Geometry check sheet. Reference: the model listing, model coordinates, mm. A direction names the side the tool comes from. Round coordinates to 2 decimals unless told otherwise and drop trailing zeros. Loops run counter-clockwise (first coordinate to the right, second up) from the corner with the lowest first, then second, coordinate; pieces in that order, holes last. Notation, with made-up numbers: M 63.25,23.5 L 115.25,23.5 A24 cw 115.25,56.5 Z; hole C 74.5,-22.75 d1. An arc over 180 degrees is marked long. Write item = value, one per line.
from build123d import *

# Parameters (mm, degrees)
SKETCH1_W           = 20
SKETCH1_H           = 20
BOSS_EXTRUDE1_DEPTH = 150
SKETCH3_R           = 9
BOSS_EXTRUDE2_DEPTH = 100
SKETCH2_R           = 7.5
BOSS_EXTRUDE3_DEPTH = 150
SKETCH7_R           = 0.25
BOSS_EXTRUDE4_DEPTH = 10
SKETCH8_R           = 2.5
BOSS_EXTRUDE5_DEPTH = 0.5
SKETCH19_W          = 126.5
SKETCH19_H          = 0.1
BOSS_EXTRUDE6_DEPTH = 0.5


with BuildPart() as part:
    # Sketch1 → Boss-Extrude1 (new body)
    with BuildSketch(Plane.XY):
        Rectangle(SKETCH1_W, SKETCH1_H)
    extrude(amount=BOSS_EXTRUDE1_DEPTH)

    # Sketch3 → Boss-Extrude2 (add)
    with BuildSketch(Plane.XZ.offset(10)):
        with Locations((0, 75)):
            Circle(SKETCH3_R)
    extrude(amount=BOSS_EXTRUDE2_DEPTH)

    # Sketch2 → Boss-Extrude3 (add)
    with BuildSketch(Plane(origin=(0, 10, 0), x_dir=(1, 0, 0), z_dir=(0, 1, 0))):
        with Locations((0, -12)):
            Circle(SKETCH2_R)
        with Locations((0, -138)):
            Circle(SKETCH2_R)
    extrude(amount=BOSS_EXTRUDE3_DEPTH)

    # Sketch7 → Boss-Extrude4 (add)
    with BuildSketch(Plane(origin=(0, 160, 0), x_dir=(1, 0, 0), z_dir=(0, 1, 0))):
        with Locations((0, -12)):
            Circle(SKETCH7_R)
        with Locations((0, -138)):
            Circle(SKETCH7_R)
    extrude(amount=BOSS_EXTRUDE4_DEPTH)

    # Sketch8 → Boss-Extrude5 (add)
    with BuildSketch(Plane(origin=(0, 170, 0), x_dir=(1, 0, 0), z_dir=(0, 1, 0))):
        with Locations((0, -12)):
            Circle(SKETCH8_R)
        with Locations((0, -138)):
            Circle(SKETCH8_R)
    extrude(amount=BOSS_EXTRUDE5_DEPTH)

    # Sketch19 → Boss-Extrude6 (add)
    with BuildSketch(Plane(origin=(0, 0, 0), x_dir=(0, 0, -1), z_dir=(1, 0, 0))):
        with Locations((-75, 164.95)):
            Rectangle(SKETCH19_W, SKETCH19_H)
    extrude(amount=BOSS_EXTRUDE6_DEPTH)


solid = part.part
(1) Sectioned sample at A-A on z = 57. Record the cut outline in (x, y), then the cut area to 3 significant figures.
Result set:
outline = M -10,-10 L 10,-10 L 10,10 L -10,10 Z; M 0,164.9 L 0.5,164.9 L 0.5,165 L 0,165 Z
area = 400 mm2
(2) Tool access check on faces 4 (the cylindrical face through (-0.33, 170.25, 135.52)), 5 (the flat face through (0, 0, 0)), 6 (the cylindrical face through (-1.951, -59.3, 66.214)). Record the directions out of +Z, -Z, +X, -X, +Y, -Y that give a thin tool (end or side, any length) a straight path to the whole face; none if there is none.
Result set:
face_4 = +Y
face_5 = -Z, +X, -X, +Y, -Y
face_6 = -Y
(3) Material ranges on line 1 along Y through (x, z) = (5, 67); line 2 along Z through (x, y) = (-1.5, 77); line 3 along Z through (x, y) = (2.5, 77), recorded low to high. Write a range as from..to.
Result set:
line_1 = -10..10
line_2 = 4.65..19.35, 130.65..145.35
line_3 = 4.93..19.07, 130.93..145.07
(4) Sectioned sample at C-C on y = 153.5. Record the cut outline in (x, z), then the cut area to 3 significant figures.
Result set:
outline = C 0,12 d15; C 0,138 d15
area = 353 mm2
(5) Sectioned sample at B-B on z = 75. Record the cut outline in (x, y), then the cut area to 3 significant figures.
Result set:
outline = M -10,-10 L -9,-10 L -9,-110 L 9,-110 L 9,-10 L 10,-10 L 10,10 L -10,10 Z; M 0,164.9 L 0.5,164.9 L 0.5,165 L 0,165 Z
area = 2,200 mm2
(6) Release check for a two-part mould opening along Y. For faces 1 (the flat face through (0, 170, 13)), 2 (the flat face through (0, 170.5, 138)), 3 (the flat face through (-10, 0, 74)) record: released by +Y, released by -Y, zero draft, split by the parting line, or undercut.
Result set:
face_1 = undercut
face_2 = released by +Y
face_3 = zero draft
(7) Depth check by flat-ended pin: pin 1 Ø10 at (x, z) = (-4, 105.5) entering from +Y; pin 2 Ø5.5 at (x, z) = (-0.5, 12) entering from -Y; pin 3 Ø5 at (x, z) = (4.5, 119.5) entering from +Y. Enter the tip coordinate at first touch or a pass-through.
Result set:
pin_1 = 165
pin_2 = -10
pin_3 = 10
